```python
from build123d import *

# Parameters (mm, degrees)
F1_DEPTH = 30
F3_DEPTH = 25


with BuildPart() as f1:
    # F0 (on Top) → F1 (new body)
    with BuildSketch(Plane.XY):
        Polygon((145, 0), (5, 0), (5, -0.974576), (118, -23), (145, -11.5), align=None)
    extrude(amount=F1_DEPTH)

    # F2 (on Front) → F3 (cut)
    with BuildSketch(Plane.XZ):
        Polygon((118, 0), (145, 0), (145, 5), align=None)
        Polygon((145, 30), (118, 30), (145, 25), align=None)
    extrude(amount=F3_DEPTH, mode=Mode.SUBTRACT)


solid = f1.part
```
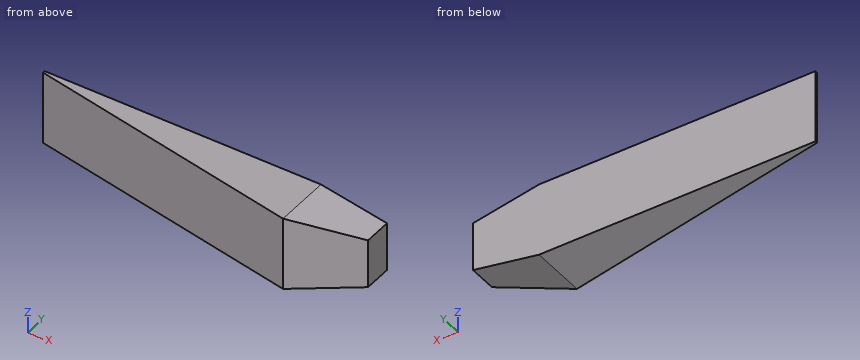
CAD build for the part. Positions are in the model's coordinates, mm. Give positions to 0.01 mm unless a question says otherwise; leave off trailing zeros. Write each loop counter-clockwise with the first axis right and the second up, starting at its lowest first coordinate (ties: lowest second). Pieces come first, ordered by that corner, then holes. Notation, with made-up numbers: M 67.5,78.5 L 120.5,78.5 A19 cw 120.5,94.5 Z; hole C 69.5,32 d7. An arc over 180 degrees is marked long. Return JSON: item names as keys, results as strings. Group by question number.
(1) Band-saw the part on C-C (x = 80). Give the cut face in (y, z), and give its area (3 significant figures).
(2) Drill centre lines: L1, parallel to Y at x = 59, z = 20.5; L2, parallel to Y at x = 83, z = 16. Where is each one in solid material? Low to high. Write a range as [from, to].
(3) Band-saw the part on B-B (y = -14.75). Give the cut face in (x, z).
(4) Flat gauge pin, fed straight in: pin 1 Ø3 at (x, y) = (120.5, -18) entering from +Z. Where does the tip first touch, or does it go through?
(5) Band-saw the part on D-D (y = -5.75). Give the cut face in (x, z), and give its area (3 significant figures).
(6) Band-saw the part on A-A (z = 19). Give the cut face in (x, y).
Entries:
{
 "1": {"outline": "M -15.59,0 L 0,0 L 0,30 L -15.59,30 Z", "area": "468 mm^2"},
 "2": {"L1": "y = [-11.5, 0]", "L2": "y = [-16.18, 0]"},
 "3": {"outline": "M 75.67,0 L 118,0 L 137.37,3.59 L 137.37,26.41 L 118,30 L 75.67,30 Z"},
 "4": {"pin 1": "stops at z = 29.81"},
 "5": {"outline": "M 29.5,0 L 118,0 L 145,5 L 145,25 L 118,30 L 29.5,30 Z", "area": "3,330 mm^2"},
 "6": {"outline": "M 5,-0.97 L 118,-23 L 145,-11.5 L 145,0 L 5,0 Z"}
}
